```python
from build123d import *

# Parameters (mm, degrees)
SKETCH_1_R               = 2.6
EXTRUDE_1_DEPTH          = 3
EXTRUDE_2_DEPTH          = 8
PATTERN_CIRCULAR_1_COUNT = 6


with BuildPart() as part:
    # Sketch 1 → Extrude 1 (new body)
    with BuildSketch(Plane(origin=(0, 0, 0), x_dir=(1, 0, 0), z_dir=(0, 1, 0))):
        Polygon((8.660254038, 15), (-8.660254038, 15), (-17.320508076, 0), (-8.660254038, -15), (8.660254038, -15), (17.320508076, 0), align=None)
        with Locations(Location((0, 0, 0), (0, 0, 270))):
            Circle(SKETCH_1_R, mode=Mode.SUBTRACT)
    extrude(amount=EXTRUDE_1_DEPTH)

    # Sketch 2 → Extrude 2 (add, symmetric)
    with BuildSketch(Plane(origin=(0, 0, 0), x_dir=(0, 0, -1), z_dir=(1, 0, 0))):
        Polygon((15, 0), (50, 0), (50, -45), (136.4, -45), (136.4, -27), (133.4, -27), (133.4, -43), (53, -43), (53, 3), (15, 3), align=None)
    extrude_2 = extrude(amount=EXTRUDE_2_DEPTH, both=True)

    # Pattern Circular 1: Extrude 2 ×6 about axis
    pattern_circular_1_axis = Axis((0, 0, 0), (0, 1, 0))
    for i in range(1, PATTERN_CIRCULAR_1_COUNT):
        add(extrude_2.rotate(pattern_circular_1_axis, i * 360 / PATTERN_CIRCULAR_1_COUNT))


solid = part.part
```
Here's how the part is built. I have some questions about the finished solid (model axes, mm). A direction names the side the tool comes from. Round coordinates to 2 decimals unless told otherwise and drop trailing zeros. Order: outer loops, then holes, each group sorted by start corner. A loop starts at its lowest first (then second) coordinate and runs counter-clockwise, first axis right, second up. Notation, with made-up numbers: M 80.25,83.5 L 109.25,83.5 A12 ccw 109.25,92.5 Z; hole C 13.5,-4 d7. An arc over 180 degrees is marked long. Answer in a Markdown table with one row per item.
Item 1: I'm going to push flat-ended pins straight in: pin 1 (16 mm diameter, centred on x = -81, z = 57, fed in from +Y); pin 2 (0.7 mm diameter, centred on x = 8, y = 1, fed in from +Z); pin 3 (1.5 mm diameter, centred on x = 1.5, z = 134.5, fed in from +Y); pin 4 (3 mm diameter, centred on x = 0, z = 0, fed in from -Y). Where does each tip first touch, or does it pass through?
A:
| item | result |
|---|---|
| pin 1 | stops at y = -43 |
| pin 2 | stops at z = 53 |
| pin 3 | stops at y = -27 |
| pin 4 | passes through |
Item 2: Imagine slicing it at C-C, the plane y = -32.5. State how many separate pieces and enclosed holes the cut face has, and give its area (3 significant figures).
A:
| item | result |
|---|---|
| separate pieces | 12 |
| enclosed holes | 0 |
| area | 576 mm2 |
Item 3: For faces 1 (the face through (0, -35, 133.4)), 2 (the face through (-45.84, -20.32, -26.6)), 3 (the face through (-115.47, -34.89, -66.8)), 4 (the face through (-117, -27, 67)), 5 (the face through (-80, -45, 46)), which set-ups out of +Z, -Z, +X, -X, +Y, -Y let a thin tool reach every point of the face, with its end or its side?
A:
| item | result |
|---|---|
| face 1 | +X, -X, +Y |
| face 2 | -Z, -X, +Y |
| face 3 | +Y |
| face 4 | +Z, -Z, +X, -X, +Y |
| face 5 | +Z, -Z, +X, -X, -Y |
Item 4: Imagine slicing it at B-B, the plane x = -86. Write out the boundary of the cut face in (y, z).
A:
| item | result |
|---|---|
| outline | M -45,-58.89 L -43,-58.89 L -43,-40.41 L -45,-40.41 Z; M -45,40.41 L -43,40.41 L -43,58.89 L -45,58.89 Z |
Item 5: Thinking about a two-plate mould opening in X: for faces 6 (the face through (81, -43, -47)), 7 (the face through (45.955, -20.322, -26.403)), 8 (the face through (-45.955, -20.322, 26.403)), 9 (the face through (-115.584, -34.888, 66.603)), which applies, +X half, -X half, draft (parallel to the pull), parting line (faces both ways), or undercut?
A:
| item | result |
|---|---|
| face 6 | undercut |
| face 7 | +X half |
| face 8 | -X half |
| face 9 | undercut |
Item 6: If I drill on L1, parallel to X at y = 0.85, z = 0; L2, parallel to X at y = -8, z = -20.5; L3, parallel to Y at x = -1.5, z = -8, over which ranges is the centre line in solid material (lowest first)? Write a range as from..to.
A:
| item | result |
|---|---|
| L1 | x = -17.32..-2.6, 2.6..17.32 |
| L2 | x = -49.36..-45.9, 45.9..49.36 |
| L3 | y = 0..3 |
Item 7: Imagine slicing it at A-A, the plane y = -7. Write out the boundary of the cut face in (x, z).
A:
| item | result |
|---|---|
| outline | M -49.9,-19.57 L -41.9,-33.43 L -39.3,-31.93 L -47.3,-18.07 Z; M -49.9,19.57 L -47.3,18.07 L -39.3,31.93 L -41.9,33.43 Z; M -8,-53 L 8,-53 L 8,-50 L -8,-50 Z; M -8,50 L 8,50 L 8,53 L -8,53 Z; M 39.3,-31.93 L 41.9,-33.43 L 49.9,-19.57 L 47.3,-18.07 Z; M 39.3,31.93 L 47.3,18.07 L 49.9,19.57 L 41.9,33.43 Z |
Item 8: Imagine slicing it at D-D, the plane z = -112. Write out the boundary of the cut face in (x, y), and give its area (3 significant figures).
A:
| item | result |
|---|---|
| outline | M -8,-45 L 8,-45 L 8,-43 L -8,-43 Z |
| area | 32.0 mm2 |
